Geometry check sheet. Reference: drawing and pictorial views, mm from the part's lowest x, y, z. Coordinates: 2 decimals unless noted, no trailing zeros. Write each loop counter-clockwise with the first axis right and the second up, starting at its lowest first coordinate (ties: lowest second). Pieces come first, ordered by that corner, then holes. Notation, with made-up numbers: M -22,75 L 27,75 A22 ccw 27,113 Z; hole C 4,9 d6. An arc over 180 degrees is marked long. One line per item, written item: value.
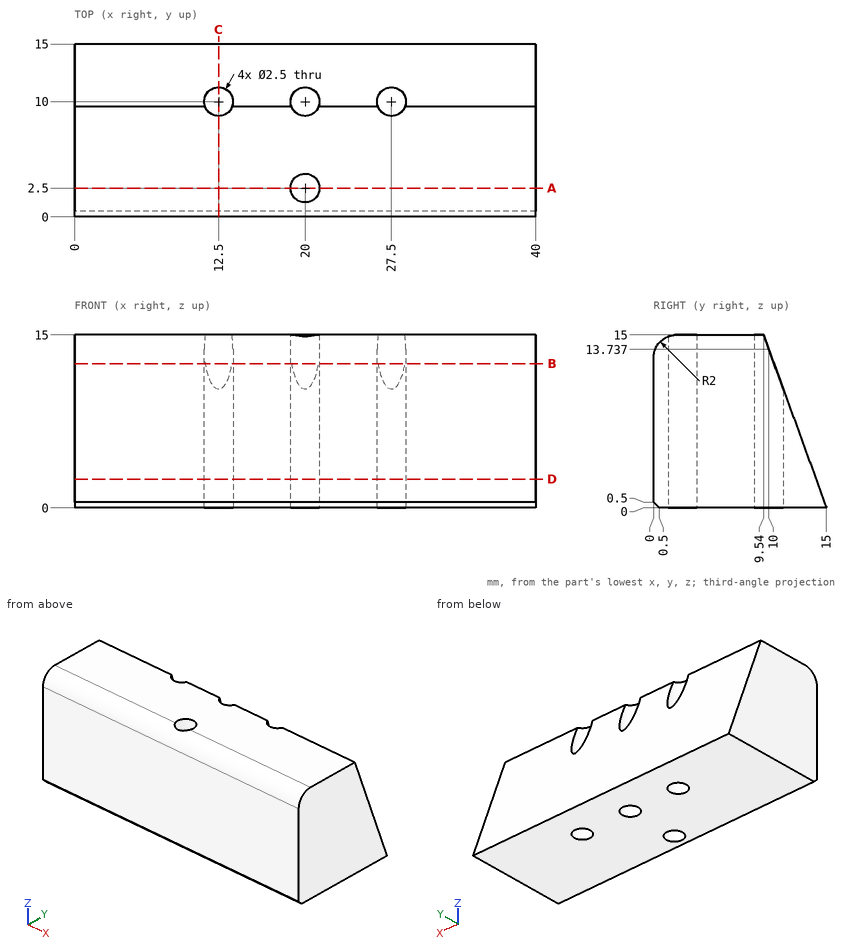
Item 1: Go/stop test with a flat-tipped pin: P1, Ø1, axis at x = 20.5, z = 8.5, coming from the +Y side. Record where the tip stops, or that it passes through.
The answers:
P1: stops at y = 12.09
Item 2: Cross-section at C-C, the plane x = 12.5. Enter the section's corners in (y, z), and give its area (3 significant figures).
The answers:
outline: M 0,0.5 L 0.5,0 L 8.75,0 L 8.75,15 L 2,15 A2 ccw 0,13 Z; M 11.25,0 L 15,0 L 11.25,10.3 Z
area: 150 mm²
Item 3: Cross-section at B-B, the plane z = 12.5. Enter the section's corners in (x, y).
The answers:
outline: M 0,0 L 40,0 L 40,10.45 L 28.67,10.45 A1.25 cw long 26.33,10.45 L 21.17,10.45 A1.25 cw long 18.83,10.45 L 13.67,10.45 A1.25 cw long 11.33,10.45 L 0,10.45 Z; hole C 20,2.5 d2.5
Item 4: Scan lines: line 1 (Y direction, x = 20, z = 11); line 2 (X direction, y = 9.25, z = 13.75); line 3 (Y direction, x = 20, z = 9.5). Record each from-to range of solid material in increasing order.
The answers:
line 1: y = 0 to 1.25, 3.75 to 8.75
line 2: x = 0 to 11.5, 13.5 to 19, 21 to 26.5, 28.5 to 40
line 3: y = 0 to 1.25, 3.75 to 8.75, 11.25 to 11.54
Item 5: Cross-section at D-D, the plane z = 2.5. Enter the section's corners in (x, y).
The answers:
outline: M 0,0 L 40,0 L 40,14.09 L 0,14.09 Z; hole C 12.5,10 d2.5; hole C 20,2.5 d2.5; hole C 20,10 d2.5; hole C 27.5,10 d2.5
Item 6: Cross-section at A-A, the plane y = 2.5. Enter the section's corners in (x, z).
The answers:
outline: M 0,0 L 18.75,0 L 18.75,15 L 0,15 Z; M 21.25,0 L 40,0 L 40,15 L 21.25,15 Z
